CAD build for the part. Positions are in the model's coordinates, mm. Face numbers are marked on the shaded views. A direction names the side the tool comes from. Coordinates: 2 decimals unless noted, no trailing zeros. Write each loop counter-clockwise with the first axis right and the second up, starting at its lowest first coordinate (ties: lowest second). Pieces come first, ordered by that corner, then holes. Notation, with made-up numbers: (73, 18.5) - (129, 18.5) arc R21 ccw to (129, 55.5) - close; hole circle Ø6 at (54, -29). An arc over 180 degrees is marked (long way). One line per question, with ' | ' between items. Start each with the question number.
1. Probe line 1 (X direction, y = -324, z = -41); line 2 (Y direction, x = -45, z = -35); line 3 (X direction, y = -31.5, z = -1). List the from-to ranges inside material, lowest first.
2. Two-plate mould, pull along Y, no slides. Class the marked faces 1, 2 and 3: +Y half, -Y half, draft (parallel to the pull), parting line (faces both ways), or undercut.
3. Band-saw the part on D-D, the plane z = 80.5. Write the cut outline in (x, y).
4. Band-saw the part on A-A, the plane z = 40. Give the number of separate pieces and of enclosed holes in the cut face, then the cut area to 3 significant figures.
5. Which spindle directions (+Z, -Z, +X, -X, +Y, -Y) get a long thin tool onto all of the face, cutting with end or side? Do the marked faces 4, 5 and 6. Say none if no direction does.
6. Band-saw the part on B-B, the plane y = -604.5. Write the cut outline in (x, z), then the cut area to 3 significant figures.
7. Band-saw the part on C-C, the plane x = 15. Write the cut outline in (y, z), then the cut area to 3 significant figures.
8. Flat gauge pins, fed straight in: P1, Ø2, axis at y = -0.5, z = -66.5, coming from the +X side; P2, Ø3, axis at x = -126.5, y = -560, coming from the +Z side; P3, Ø8.5, axis at x = 204.5, y = -332.5, coming from the +Z side. Where does each tip first touch, or does it go through?
from build123d import *

# Parameters (mm, degrees)
F0_W     = 32
F0_H     = 20
F1_DEPTH = 650
F2_T     = -2.5
F3_D     = 115
F4_DEPTH = 25


with BuildPart() as f1:
    # F0 (on Front) → F1 (new body)
    with BuildSketch(Plane.XZ):
        Polygon((217.8639564514, 95.5699048042), (-222.1360435486, 95.5699048042), (-222.1360435486, -24.4300951958), (-205.1360435486, -24.4300951958), (-205.1360435486, -84.4300951958), (200.8639564514, -84.4300951958), (200.8639564514, -24.4300951958), (217.8639564514, -24.4300951958), align=None)
        with Locations((-174.1360435486, -65.4300951958)):
            Rectangle(F0_W, F0_H, mode=Mode.SUBTRACT)
    extrude(amount=F1_DEPTH)

    # F2
    f2_openings = [f1.faces().sort_by_distance(p)[0] for p in [
        (-2.136044, -325, 95.569905),
    ]]
    offset(amount=F2_T, openings=f2_openings, kind=Kind.INTERSECTION)

    # F3 (through all)
    with Locations(Plane(origin=(0, 0, 0), x_dir=(1, 0, 0), z_dir=(0, 1, 0))):
        with Locations((-132.1360435486, -5.5699048042), (-2.1360435486, -5.5699048042), (127.8639564514, -5.5699048042)):
            Hole(F3_D / 2)

    # F4 (cut): a face of the model
    f4_faces = [f1.faces().sort_by_distance(p)[0] for p in [
        (-174.1360435486, -325, -52.9300951958),
    ]]
    extrude(f4_faces, amount=-F4_DEPTH, mode=Mode.SUBTRACT)


solid = f1.part
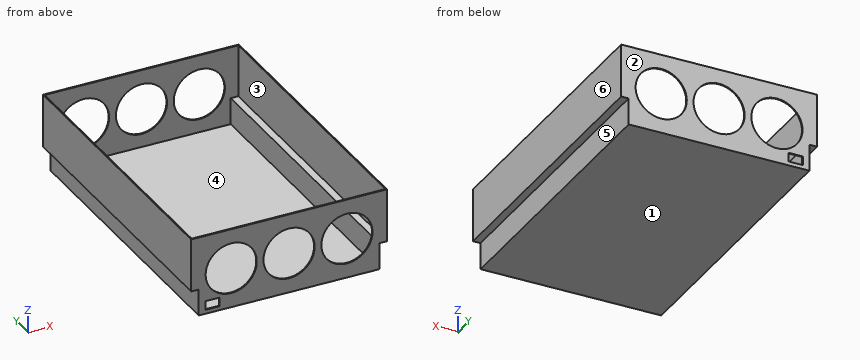
Filled in:
1) line 1: x = -205.14 to -202.64, 198.36 to 200.86 | line 2: y = -650 to -647.5, -2.5 to 0 | line 3: x = -222.14 to -219.64, 215.36 to 217.86
2) face 1: draft | face 2: +Y half | face 3: undercut
3) outline: (-222.14, -650) - (217.86, -650) - (217.86, 0) - (-222.14, 0) - close; hole (-219.64, -647.5) - (215.36, -647.5) - (215.36, -2.5) - (-219.64, -2.5) - close
4) separate pieces: 6 | enclosed holes: 0 | area: 4,040 mm²
5) face 4: +Z | face 5: -Z, +X, +Y, -Y | face 6: +Z, -Z, +X, +Y, -Y
6) outline: (-222.14, -24.43) - (-205.14, -24.43) - (-205.14, -84.43) - (200.86, -84.43) - (200.86, -24.43) - (217.86, -24.43) - (217.86, 95.57) - (215.36, 95.57) - (215.36, -21.93) - (198.36, -21.93) - (198.36, -81.93) - (-202.64, -81.93) - (-202.64, -21.93) - (-219.64, -21.93) - (-219.64, 95.57) - (-222.14, 95.57) - close | area: 1,990 mm²
7) outline: (-650, -84.43) - (0, -84.43) - (0, -49.32) - (-2.5, -49.32) - (-2.5, -81.93) - (-647.5, -81.93) - (-647.5, -49.32) - (-650, -49.32) - close; (-650, 60.46) - (-647.5, 60.46) - (-647.5, 95.57) - (-650, 95.57) - close; (-2.5, 60.46) - (0, 60.46) - (0, 95.57) - (-2.5, 95.57) - close | area: 1,960 mm²
8) P1: stops at x = 200.86 | P2: stops at z = -81.93 | P3: stops at z = -21.93
